from build123d import *

# Parameters (mm, degrees)
CROQUIS1_W                          = 50.8
CROQUIS1_H                          = 38.5191
SALIENTE_EXTRUIR1_DEPTH             = 7.366
CORTAR_EXTRUIR1_DEPTH               = 55.825434081
TALADROS_DE_ESPIGA_DE_5_16_0_28_1_D = 7.112
CORTAR_EXTRUIR2_DEPTH               = 33.167303123
TALADRO_ROSCADO_10_241_D            = 3.7973


with BuildPart() as part:
    # Croquis1 → Saliente-Extruir1 (new body)
    with BuildSketch(Plane(origin=(0, 0, 0), x_dir=(1, 0, 0), z_dir=(0, 1, 0))):
        Rectangle(CROQUIS1_W, CROQUIS1_H)
    extrude(amount=SALIENTE_EXTRUIR1_DEPTH)

    # Croquis2 → Cortar-Extruir1 (cut, through all)
    with BuildSketch(Plane(origin=(25.4, 0, 0), x_dir=(0, 0, -1), z_dir=(1, 0, 0))):
        Polygon((19.25955, 3.048), (12.90955, 3.048), (12.90955, 6.35), (-0.17145, 6.35), (-0.17145, 7.366), (19.25955, 7.366), align=None)
    extrude(amount=-CORTAR_EXTRUIR1_DEPTH, mode=Mode.SUBTRACT)

    # Taladros de espiga de 5/16 (0.28)1 (through all)
    with Locations(Plane(origin=(0, 7.366, 0), x_dir=(1, 0, 0), z_dir=(0, 1, 0))):
        with Locations((17.4625, -11.32205), (0, -11.32205), (-17.4625, -11.32205)):
            Hole(TALADROS_DE_ESPIGA_DE_5_16_0_28_1_D / 2)

    # Croquis5 → Cortar-Extruir2 (cut, through all)
    with BuildSketch(Plane(origin=(0, 3.048, 0), x_dir=(1, 0, 0), z_dir=(0, 1, 0))):
        Polygon((-2.2225, 19.25955), (-1.27, 17.78635), (1.27, 17.78635), (2.2225, 19.25955), align=None)
    extrude(amount=-CORTAR_EXTRUIR2_DEPTH, mode=Mode.SUBTRACT)

    # Taladro roscado #10-241 (through all)
    with Locations(Plane(origin=(0, 6.35, 0), x_dir=(1, 0, 0), z_dir=(0, 1, 0))):
        with Locations((19.05, 6.55955), (0, 6.55955), (-19.05, 6.55955)):
            Hole(TALADRO_ROSCADO_10_241_D / 2)


solid = part.part
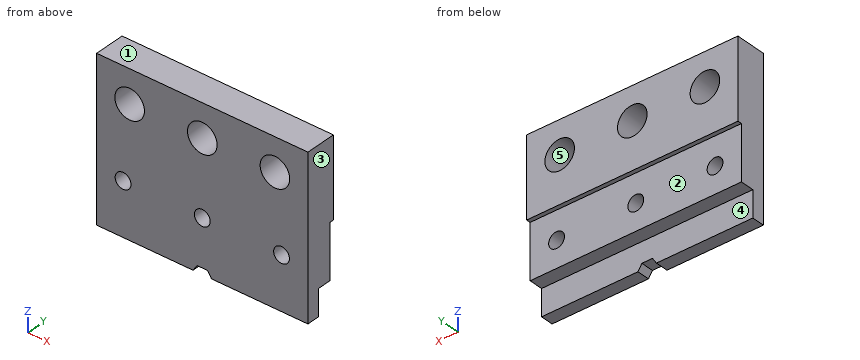
Read the model definition and answer for the solid it produces. Units are mm, in the model's axes. Face numbers are marked on the shaded views. A direction names the side the tool comes from. Coordinates: 2 decimals unless noted, no trailing zeros. Loops run counter-clockwise (first coordinate to the right, second up) from the corner with the lowest first, then second, coordinate; pieces in that order, holes last. Notation, with made-up numbers: (-35.5, 85) -> (12.5, 85) arc R26 cw to (12.5, 119) -> close; hole circle Ø5 at (-35, 9.25). An arc over 180 degrees is marked (long way). Write item = value, one per line. Start each with the question number.
1) The mould has two halves that part along X. Classify the marked faces 3, 4 and 5: pulls with the +X half, pulls with the -X half, needs draft (parallel to the pull), parting line crosses it, or undercut.
2) The part is cut by section D-D, the plane x = -9.5. Determine the outline of the cut face in (y, z).
3) Given P1, Ø14.5, axis at x = 7, z = -5, coming from the +Y side; P2, Ø1.3, axis at x = -0.5, y = 1, coming from the -Z side; P3, Ø7, axis at x = -6, z = -16, coming from the +Y side; P4, Ø2, axis at x = 12, y = 5, coming from the -Z side, each flat-ended and moving along its own axis, determine where each tip first touches the part or whether it passes through.
4) Find the intervals of material crossed by L1, parallel to Z at x = 0, y = 1.75; L2, parallel to Z at x = 0, y = 3.5; L3, parallel to X at y = 1.25, z = 12, in increasing order. Write a range as from..to.
5) The part is cut by section B-B, the plane y = 2.5. Determine the outline of the cut face in (x, z).
6) For the marked faces 1 and 2, determine the directions among +Z, -Z, +X, -X, +Y, -Y from which every point of the face is accessible in a straight line to the end or side of a thin tool.
7) The part is cut by section C-C, the plane z = 9. Determine the outline of the cut face in (x, y).
8) The part is cut by section A-A, the plane x = 0. Determine the outline of the cut face in (y, z).
Result:
q1.face_3 = pulls with the +X half
q1.face_4 = needs draft
q1.face_5 = undercut
q2.outline = (0, -19.26) -> (3.05, -19.26) -> (3.05, -12.91) -> (6.35, -12.91) -> (6.35, 0.17) -> (7.37, 0.17) -> (7.37, 19.26) -> (0, 19.26) -> close
q3.P1 = 7.37
q3.P2 = -17.79
q3.P3 = 6.35
q3.P4 = -12.91
q4.L1 = -17.79..-8.46, -4.66..7.77, 14.88..19.26
q4.L2 = -12.91..-8.46, -4.66..7.77, 14.88..19.26
q4.L3 = -25.4..-20.95, -13.97..-3.49, 3.49..13.97, 20.95..25.4
q5.outline = (-25.4, -19.26) -> (-2.22, -19.26) -> (-1.27, -17.79) -> (1.27, -17.79) -> (2.22, -19.26) -> (25.4, -19.26) -> (25.4, 19.26) -> (-25.4, 19.26) -> close; hole circle Ø7.11 at (-17.46, 11.32); hole circle Ø3.8 at (-19.05, -6.56); hole circle Ø7.11 at (0, 11.32); hole circle Ø3.8 at (0, -6.56); hole circle Ø7.11 at (17.46, 11.32); hole circle Ø3.8 at (19.05, -6.56)
q6.face_1 = +Z, +X, -X, +Y, -Y
q6.face_2 = -Z, +X, -X, +Y
q7.outline = (-25.4, 0) -> (-20.16, 0) -> (-20.16, 7.37) -> (-25.4, 7.37) -> close; (-14.77, 0) -> (-2.69, 0) -> (-2.69, 7.37) -> (-14.77, 7.37) -> close; (2.69, 0) -> (14.77, 0) -> (14.77, 7.37) -> (2.69, 7.37) -> close; (20.16, 0) -> (25.4, 0) -> (25.4, 7.37) -> (20.16, 7.37) -> close
q8.outline = (0, -17.79) -> (3.05, -17.79) -> (3.05, -12.91) -> (6.35, -12.91) -> (6.35, -8.46) -> (0, -8.46) -> close; (0, -4.66) -> (6.35, -4.66) -> (6.35, 0.17) -> (7.37, 0.17) -> (7.37, 7.77) -> (0, 7.77) -> close; (0, 14.88) -> (7.37, 14.88) -> (7.37, 19.26) -> (0, 19.26) -> close
